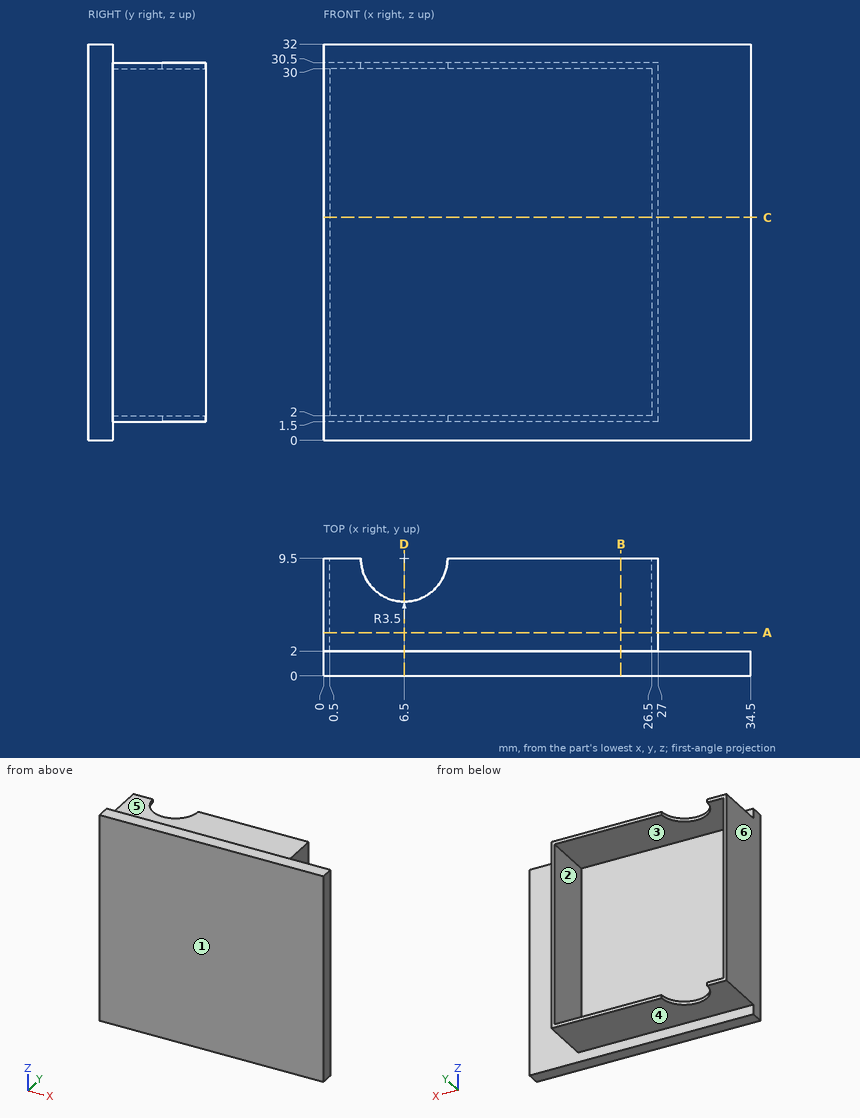
Print and shaded views of the part. All mm, measured from the part's lowest x, y and z. A direction names the side the tool comes from. Give positions to 0.01 mm unless a question says otherwise; leave off trailing zeros. Loops run counter-clockwise (first coordinate to the right, second up) from the corner with the lowest first, then second, coordinate; pieces in that order, holes last. Notation, with made-up numbers: (-18, 88) -> (32, 88) arc R15 ccw to (32, 107) -> close; hole circle Ø4 at (-16, 21). An arc over 180 degrees is marked (long way). One line per question, with ' | ' between items. Start each with the question number.
1) Two-plate mould, pull along Z, no slides. Class the marked faces 3, 4, 5 and 6: released by +Z, released by -Z, zero draft, split by the parting line, or undercut.
2) Cut at B-B (x = 24). Give the cut face in (y, z).
3) Cut at C-C (z = 18). Give the cut face in (x, y).
4) Pin check, flat tips, straight feed: pin 1 (2 mm diameter, centred on y = 4.5, z = 28, fed in from +X); pin 2 (13 mm diameter, centred on x = 17, z = 9.5, fed in from +Y); pin 3 (3 mm diameter, centred on x = 13.5, y = 6, fed in from -Z). Stop position of each tip, or through.
5) Cut at A-A (y = 3.5). Give the cut face in (x, z), plus the area to 3 significant figures.
6) Cut at D-D (x = 6.5). Give the cut face in (y, z), plus the area to 3 significant figures.
7) Probe L1, parallel to X at y = 9, z = 5; L2, parallel to Z at x = 21, y = 5.25; L3, parallel to Y at x = 6.5, z = 16. List the from-to ranges inside material, lowest first.
8) 3-axis set-ups, long thin cutter, end or side, ignore diameter. For the marked faces 1 and 2: which of +Z, -Z, +X, -X, +Y, -Y reach the whole face in a straight line?
Return value:
1) face 3: undercut | face 4: released by -Z | face 5: released by +Z | face 6: zero draft
2) outline: (0, 0) -> (2, 0) -> (2, 1.5) -> (9.5, 1.5) -> (9.5, 2) -> (2, 2) -> (2, 30) -> (9.5, 30) -> (9.5, 30.5) -> (2, 30.5) -> (2, 32) -> (0, 32) -> close
3) outline: (0, 0) -> (34.5, 0) -> (34.5, 2) -> (27, 2) -> (27, 9.5) -> (26.5, 9.5) -> (26.5, 2) -> (0.5, 2) -> (0.5, 9.5) -> (0, 9.5) -> close
4) pin 1: x = 27 | pin 2: y = 2 | pin 3: z = 1.5
5) outline: (0, 1.5) -> (27, 1.5) -> (27, 30.5) -> (0, 30.5) -> close; hole (0.5, 2) -> (26.5, 2) -> (26.5, 30) -> (0.5, 30) -> close | area: 55.0 mm^2
6) outline: (0, 0) -> (2, 0) -> (2, 1.5) -> (6, 1.5) -> (6, 2) -> (2, 2) -> (2, 30) -> (6, 30) -> (6, 30.5) -> (2, 30.5) -> (2, 32) -> (0, 32) -> close | area: 68.0 mm^2
7) L1: 0 to 0.5, 26.5 to 27 | L2: 1.5 to 2, 30 to 30.5 | L3: 0 to 2
8) face 1: +Z, -Z, +X, -X, -Y | face 2: +Y
